The listing builds one solid part. Answer for the finished solid, in the listing's coordinates (mm). A direction names the side the tool comes from. Give positions to 0.01 mm unless a question says otherwise; leave off trailing zeros. Loops run counter-clockwise (first coordinate to the right, second up) from the corner with the lowest first, then second, coordinate; pieces in that order, holes last. Notation, with made-up numbers: (43, -6.75) -> (99, -6.75) arc R19 cw to (99, 20.25) -> close; hole circle Ø11 at (4.25, 10.25). An arc over 180 degrees is marked (long way). One line per question, with ' | ' between items. Start each with the question number.
Autodesk Inventor part; units mm, degrees
ref_plane "YZ Plane" through (0, 0, 0) normal (1, 0, 0) x (0, 1, 0)
ref_plane "XZ Plane" through (0, 0, 0) normal (0, 1, 0) x (-1, 0, 0)
ref_plane "XY Plane" through (0, 0, 0) normal (0, 0, 1) x (1, 0, 0)
sketch "Esboço2" plane through (0, 0, 0) normal (0, 0, 1) x (1, 0, 0)
  line L0 (0, 0) -> (9.5, 0)
  line L1 (9.5, 0) -> (9.5, 9.8)
  line L2 (9.5, 9.8) -> (0, 9.8)
  line L3 (0, 9.8) -> (0, 0)
  dimension "d0" = 9.5
  dimension "d1" = 9.8
revolve "Revolução1" add sketch "Esboço2" angle 360 about axis through (0, 0, 0) along (1, 0, 0)
sketch "Esboço3" plane through (0, 0, 0) normal (-1, 0, 0) x (0, 0, 1)
  circle A0 centre (0, 0) radius 1.75
  dimension "d3" = 3.5
extrude "Extrusão1" cut sketch "Esboço3" against normal blind 4.85
sketch "Esboço4" plane through (0, 0, 0) normal (-1, 0, 0) x (0, 0, 1)
  circle A0 centre (0, 0) radius 4.5
  dimension "d6" = 9
extrude "Extrusão2" cut sketch "Esboço4" against normal blind 2
sketch "Esboço11" plane through (9.5, 0, 0) normal (1, 0, 0) x (0, 0, -1)
  circle A0 centre (0, 0) radius 2.55
  circle A1 centre (0, 0) radius 2.95
  line L0 (0, 0) -> (2.95, 0)
  line L1 (2.55, 0) -> (2.5493, 0.06)
  line L2 (2.5493, 0.06) -> (2.55, 0)
  line L3 (2.55, 0) -> (2.5493, -0.06)
  line L4 (2.5493, 0.06) -> (2.9315, 0.3295)
  line L5 (2.5493, -0.06) -> (2.9315, -0.3295)
  line L6 (2.9315, 0.3295) -> (2.9255, 0.3791)
  line L7 (2.9315, -0.3295) -> (2.9255, -0.3791)
  line L8 (2.406, 0.8448) -> (2.6862, 1.2193)
  line L9 (2.4252, 0.788) -> (2.406, 0.8448)
  line L10 (2.4252, 0.788) -> (2.4431, 0.7307)
  line L11 (2.4431, 0.7307) -> (2.8899, 0.5925)
  circle A2 centre (0, 0) radius 2.95
  line L12 (2.6862, 1.2193) -> (2.6652, 1.2646)
  line L13 (2.8899, 0.5925) -> (2.8995, 0.5435)
  line L14 (2.0272, 1.547) -> (2.178, 1.9897)
  line L15 (2.063, 1.4989) -> (2.0272, 1.547)
  line L16 (2.063, 1.4989) -> (2.0977, 1.4499)
  line L17 (2.0977, 1.4499) -> (2.5653, 1.4566)
  circle A3 centre (0, 0) radius 2.95
  line L18 (2.178, 1.9897) -> (2.144, 2.0263)
  line L19 (2.5653, 1.4566) -> (2.5897, 1.4129)
  line L20 (1.4499, 2.0977) -> (1.4566, 2.5653)
  line L21 (1.4989, 2.063) -> (1.4499, 2.0977)
  line L22 (1.4989, 2.063) -> (1.547, 2.0272)
  line L23 (1.547, 2.0272) -> (1.9897, 2.178)
  circle A4 centre (0, 0) radius 2.95
  line L24 (1.4566, 2.5653) -> (1.4129, 2.5897)
  line L25 (1.9897, 2.178) -> (2.0263, 2.144)
  line L26 (0.7307, 2.4431) -> (0.5925, 2.8899)
  line L27 (0.788, 2.4252) -> (0.7307, 2.4431)
  line L28 (0.788, 2.4252) -> (0.8448, 2.406)
  line L29 (0.8448, 2.406) -> (1.2193, 2.6862)
  circle A5 centre (0, 0) radius 2.95
  line L30 (0.5925, 2.8899) -> (0.5435, 2.8995)
  line L31 (1.2193, 2.6862) -> (1.2646, 2.6652)
  line L32 (-0.06, 2.5493) -> (-0.3295, 2.9315)
  line L33 (0, 2.55) -> (-0.06, 2.5493)
  line L34 (0, 2.55) -> (0.06, 2.5493)
  line L35 (0.06, 2.5493) -> (0.3295, 2.9315)
  circle A6 centre (0, 0) radius 2.95
  line L36 (-0.3295, 2.9315) -> (-0.3791, 2.9255)
  line L37 (0.3295, 2.9315) -> (0.3791, 2.9255)
  line L38 (-0.8448, 2.406) -> (-1.2193, 2.6862)
  line L39 (-0.788, 2.4252) -> (-0.8448, 2.406)
  line L40 (-0.788, 2.4252) -> (-0.7307, 2.4431)
  line L41 (-0.7307, 2.4431) -> (-0.5925, 2.8899)
  circle A7 centre (0, 0) radius 2.95
  line L42 (-1.2193, 2.6862) -> (-1.2646, 2.6652)
  line L43 (-0.5925, 2.8899) -> (-0.5435, 2.8995)
  line L44 (-1.547, 2.0272) -> (-1.9897, 2.178)
  line L45 (-1.4989, 2.063) -> (-1.547, 2.0272)
  line L46 (-1.4989, 2.063) -> (-1.4499, 2.0977)
  line L47 (-1.4499, 2.0977) -> (-1.4566, 2.5653)
  circle A8 centre (0, 0) radius 2.95
  line L48 (-1.9897, 2.178) -> (-2.0263, 2.144)
  line L49 (-1.4566, 2.5653) -> (-1.4129, 2.5897)
  line L50 (-2.0977, 1.4499) -> (-2.5653, 1.4566)
  line L51 (-2.063, 1.4989) -> (-2.0977, 1.4499)
  line L52 (-2.063, 1.4989) -> (-2.0272, 1.547)
  line L53 (-2.0272, 1.547) -> (-2.178, 1.9897)
  circle A9 centre (0, 0) radius 2.95
  line L54 (-2.5653, 1.4566) -> (-2.5897, 1.4129)
  line L55 (-2.178, 1.9897) -> (-2.144, 2.0263)
  line L56 (-2.4431, 0.7307) -> (-2.8899, 0.5925)
  line L57 (-2.4252, 0.788) -> (-2.4431, 0.7307)
  line L58 (-2.4252, 0.788) -> (-2.406, 0.8448)
  line L59 (-2.406, 0.8448) -> (-2.6862, 1.2193)
  circle A10 centre (0, 0) radius 2.95
  line L60 (-2.8899, 0.5925) -> (-2.8995, 0.5435)
  line L61 (-2.6862, 1.2193) -> (-2.6652, 1.2646)
  line L62 (-2.5493, -0.06) -> (-2.9315, -0.3295)
  line L63 (-2.55, 0) -> (-2.5493, -0.06)
  line L64 (-2.55, 0) -> (-2.5493, 0.06)
  line L65 (-2.5493, 0.06) -> (-2.9315, 0.3295)
  circle A11 centre (0, 0) radius 2.95
  line L66 (-2.9315, -0.3295) -> (-2.9255, -0.3791)
  line L67 (-2.9315, 0.3295) -> (-2.9255, 0.3791)
  line L68 (-2.406, -0.8448) -> (-2.6862, -1.2193)
  line L69 (-2.4252, -0.788) -> (-2.406, -0.8448)
  line L70 (-2.4252, -0.788) -> (-2.4431, -0.7307)
  line L71 (-2.4431, -0.7307) -> (-2.8899, -0.5925)
  circle A12 centre (0, 0) radius 2.95
  line L72 (-2.6862, -1.2193) -> (-2.6652, -1.2646)
  line L73 (-2.8899, -0.5925) -> (-2.8995, -0.5435)
  line L74 (-2.0272, -1.547) -> (-2.178, -1.9897)
  line L75 (-2.063, -1.4989) -> (-2.0272, -1.547)
  line L76 (-2.063, -1.4989) -> (-2.0977, -1.4499)
  line L77 (-2.0977, -1.4499) -> (-2.5653, -1.4566)
  circle A13 centre (0, 0) radius 2.95
  line L78 (-2.178, -1.9897) -> (-2.144, -2.0263)
  line L79 (-2.5653, -1.4566) -> (-2.5897, -1.4129)
  line L80 (-1.4499, -2.0977) -> (-1.4566, -2.5653)
  line L81 (-1.4989, -2.063) -> (-1.4499, -2.0977)
  line L82 (-1.4989, -2.063) -> (-1.547, -2.0272)
  line L83 (-1.547, -2.0272) -> (-1.9897, -2.178)
  circle A14 centre (0, 0) radius 2.95
  line L84 (-1.4566, -2.5653) -> (-1.4129, -2.5897)
  line L85 (-1.9897, -2.178) -> (-2.0263, -2.144)
  line L86 (-0.7307, -2.4431) -> (-0.5925, -2.8899)
  line L87 (-0.788, -2.4252) -> (-0.7307, -2.4431)
  line L88 (-0.788, -2.4252) -> (-0.8448, -2.406)
  line L89 (-0.8448, -2.406) -> (-1.2193, -2.6862)
  circle A15 centre (0, 0) radius 2.95
  line L90 (-0.5925, -2.8899) -> (-0.5435, -2.8995)
  line L91 (-1.2193, -2.6862) -> (-1.2646, -2.6652)
  line L92 (0.06, -2.5493) -> (0.3295, -2.9315)
  line L93 (0, -2.55) -> (0.06, -2.5493)
  line L94 (0, -2.55) -> (-0.06, -2.5493)
  line L95 (-0.06, -2.5493) -> (-0.3295, -2.9315)
  circle A16 centre (0, 0) radius 2.95
  line L96 (0.3295, -2.9315) -> (0.3791, -2.9255)
  line L97 (-0.3295, -2.9315) -> (-0.3791, -2.9255)
  line L98 (0.8448, -2.406) -> (1.2193, -2.6862)
  line L99 (0.788, -2.4252) -> (0.8448, -2.406)
  line L100 (0.788, -2.4252) -> (0.7307, -2.4431)
  line L101 (0.7307, -2.4431) -> (0.5925, -2.8899)
  circle A17 centre (0, 0) radius 2.95
  line L102 (1.2193, -2.6862) -> (1.2646, -2.6652)
  line L103 (0.5925, -2.8899) -> (0.5435, -2.8995)
  line L104 (1.547, -2.0272) -> (1.9897, -2.178)
  line L105 (1.4989, -2.063) -> (1.547, -2.0272)
  line L106 (1.4989, -2.063) -> (1.4499, -2.0977)
  line L107 (1.4499, -2.0977) -> (1.4566, -2.5653)
  circle A18 centre (0, 0) radius 2.95
  line L108 (1.9897, -2.178) -> (2.0263, -2.144)
  line L109 (1.4566, -2.5653) -> (1.4129, -2.5897)
  line L110 (2.0977, -1.4499) -> (2.5653, -1.4566)
  line L111 (2.063, -1.4989) -> (2.0977, -1.4499)
  line L112 (2.063, -1.4989) -> (2.0272, -1.547)
  line L113 (2.0272, -1.547) -> (2.178, -1.9897)
  circle A19 centre (0, 0) radius 2.95
  line L114 (2.5653, -1.4566) -> (2.5897, -1.4129)
  line L115 (2.178, -1.9897) -> (2.144, -2.0263)
  line L116 (2.4431, -0.7307) -> (2.8899, -0.5925)
  line L117 (2.4252, -0.788) -> (2.4431, -0.7307)
  line L118 (2.4252, -0.788) -> (2.406, -0.8448)
  line L119 (2.406, -0.8448) -> (2.6862, -1.2193)
  circle A20 centre (0, 0) radius 2.95
  line L120 (2.8899, -0.5925) -> (2.8995, -0.5435)
  line L121 (2.6862, -1.2193) -> (2.6652, -1.2646)
  point P0 (2.8056, 0.9116)
  point P1 (2.3866, 1.734)
  point P2 (1.734, 2.3866)
  point P3 (0.9116, 2.8056)
  point P4 (0, 2.95)
  point P5 (-0.9116, 2.8056)
  point P6 (-1.734, 2.3866)
  point P7 (-2.3866, 1.734)
  point P8 (-2.8056, 0.9116)
  point P9 (-2.95, 0)
  point P10 (-2.8056, -0.9116)
  point P11 (-2.3866, -1.734)
  point P12 (-1.734, -2.3866)
  point P13 (-0.9116, -2.8056)
  point P14 (0, -2.95)
  point P15 (0.9116, -2.8056)
  point P16 (1.734, -2.3866)
  point P17 (2.3866, -1.734)
  point P18 (2.8056, -0.9116)
  dimension "d59" = 5.9
  dimension "d58" = 5.1
  dimension "d60" = 0.06
  dimension "d61" = 0.06
  dimension "d62" = 0.05
  dimension "d63" = 0.05
  dimension "d66" = 360
extrude "Extrusão5" cut sketch "Esboço11" against normal blind 3.5 contours A0 | A0 L11 A1 L4 | L5 A1 L116 A0 | A0 L17 A1 L8 | L119 A1 L110 A0 | A0 L23 A1 L14 | L113 A1 L104 A0 | A0 L29 A1 L20 | L107 A1 L98 A0 | A0 L35 A1 L26 | L101 A1 L92 A0 | A0 L41 A1 L32 | L95 A1 L86 A0 | A0 L47 A1 L38 | L89 A1 L80 A0 | A0 L53 A1 L44 | L83 A1 L74 A0 | A0 L59 A1 L50 | L77 A1 L68 A0 | A0 L65 A1 L56 | L71 A1 L62 A0
sketch "Esboço12" plane through (9.5, 0, 0) normal (1, 0, 0) x (0, 0, -1)
  point P0 (0, 0)
properties part number "roda certa 2.0"
1. The part is cut by section A-A (x = 0.75). Write down the section's boundary in (y, z).
2. The part is cut by section D-D (x = 4). Write down the section's boundary in (y, z), plus the area to 3 significant figures.
3. Straight lines are drawn through the part: L1, parallel to Z at x = 4.5, y = 1.25; L2, parallel to Z at x = 1.5, y = -2; L3, parallel to X at y = -3.5, z = 2.75. For each, find the intervals that lie inside material, in ascending order.
4. The part is cut by section B-B (y = -4). Write down the section's boundary in (x, z).
5. For faces 1 (the flat face through (9.5, -2.3, 2.3)), 2 (the flat face through (6, 0, 0)), 3 (the flat face through (2, -2, 0)), determine the directions among +Z, -Z, +X, -X, +Y, -Y from which every point of the face is accessible in a straight line to the end or side of a thin tool.
6. The part is cut by section C-C (z = 8). Write down the section's boundary in (x, y), plus the area to 3 significant figures.
7. Determine the mould class of faces 4 (the cylindrical face through (3.405, -0.67, 1.617)), 5 (the cylindrical face through (4.684, -2.124, 9.567)), 6 (the flat face through (0, 4.2, -2)) for opening direction Y: released by +Y, released by -Y, zero draft, split by the parting line, or undercut.
8. Each of these flat-tipped pins is pushed along its axis until it touches: pin 1 Ø4 at (y, z) = (0, 0) entering from +X; pin 2 Ø4 at (y, z) = (0, -0.5) entering from -X; pin 3 Ø2 at (y, z) = (0, -0.5) entering from -X. Where does it stop, or does it pass through?
Check sheet entries:
1) outline: circle Ø19.6 at (0, 0); hole circle Ø9 at (0, 0)
2) outline: circle Ø19.6 at (0, 0); hole circle Ø3.5 at (0, 0) | area: 292 mm^2
3) L1: z = -9.72 to -1.22, 1.22 to 9.72 | L2: z = -9.59 to -4.03, 4.03 to 9.59 | L3: x = 2 to 9.5
4) outline: (0, -8.95) -> (9.5, -8.95) -> (9.5, 8.95) -> (0, 8.95) -> (0, 2.06) -> (2, 2.06) -> (2, -2.06) -> (0, -2.06) -> close
5) face 1: +Z, -Z, +X, +Y, -Y | face 2: +X | face 3: -X
6) outline: (0, -5.66) -> (9.5, -5.66) -> (9.5, 5.66) -> (0, 5.66) -> close | area: 108 mm^2
7) face 4: undercut | face 5: split by the parting line | face 6: zero draft
8) pin 1: stops at x = 6 | pin 2: stops at x = 2 | pin 3: stops at x = 4.85
